Can you work these out from the model? Positions are in its coordinate system, mm. Give positions to 0.01 mm unless a question says otherwise; leave off trailing zeros. Order: outer loops, then holes, each group sorted by start corner. A loop starts at its lowest first (then second) coordinate and runs counter-clockwise, first axis right, second up. Notation, with made-up numbers: M 2.5,16 L 28.5,16 A17 ccw 28.5,41 Z; hole C -32,43.25 d8. An arc over 180 degrees is marked long. Answer as a JSON object with one key per item and string values.
Autodesk Inventor part; units mm, degrees
ref_plane "YZ Plane" through (0, 0, 0) normal (1, 0, 0) x (0, 1, 0)
ref_plane "XZ Plane" through (0, 0, 0) normal (0, 1, 0) x (-1, 0, 0)
ref_plane "XY Plane" through (0, 0, 0) normal (0, 0, 1) x (1, 0, 0)
sketch "Sketch1" plane through (0, 0, 0) normal (0, 0, 1) x (1, 0, 0)
  circle A0 centre (0, 0) radius 8.001
  dimension "d0" = 16.002
extrude "Extrusion1" add sketch "Sketch1" along normal mid plane 20.574
sketch "Sketch2" plane through (0, 0, 10.287) normal (0, 0, 1) x (1, 0, 0)
  circle A0 centre (0, 0) radius 8.001
  circle A1 centre (0, 0) radius 14.351
  dimension "d29" = 28.702
extrude "Extrusion2" add sketch "Sketch2" along normal blind 4.826 contours A0 | A1
sketch "Sketch4" plane through (0, 0, -10.287) normal (0, 0, -1) x (-1, 0, 0)
  circle A0 centre (0, 0) radius 8.001
hole "Hole2" at (0, 0, -10.287) direction (0, 0, 1) diameter 7.7978 end through all
chamfer "Chamfer1" distance 0.381 angle 45 1 edges at (-8.001, 0, -10.287)
sketch "Sketch6" plane through (0, 0, 15.113) normal (0, 0, 1) x (1, 0, 0)
  circle A0 centre (0, 0) radius 14.351
  circle A1 centre (0, 0) radius 11.4134 construction
  point P0 (0, 11.4134)
hole "Hole3" at (0, 11.4134, 15.113) direction (0, 0, -1) diameter 3.556 end through all
pattern_circular "Circular Pattern1" count 3 over 360 about axis through (0, 0, 10.287) along (0, 0, 1) of "Hole3"
properties part number "LeadScrewNut" material "ABS Plastic"
1) I'm going to push flat-ended pins straight in: pin 1 Ø1 at (x, z) = (-3, 9) entering from +Y; pin 2 Ø4 at (y, z) = (4, -2) entering from -X; pin 3 Ø6 at (y, z) = (-3, 7.5) entering from -X. Where does each tip first touch, or does it pass through?
Results found:
{"pin 1": "stops at y = 7.6", "pin 2": "stops at x = -7.75", "pin 3": "stops at x = -14.23"}
2) I want a section at A-A on y = 0. Write out the boundary of the cut face in (x, z).
Results found:
{"outline": "M -14.35,10.29 L -8,10.29 L -8,-9.91 L -7.62,-10.29 L -3.9,-10.29 L -3.9,15.11 L -14.35,15.11 Z; M 3.9,-10.29 L 7.62,-10.29 L 8,-9.91 L 8,10.29 L 14.35,10.29 L 14.35,15.11 L 3.9,15.11 Z"}
3) I want a section at B-B on x = 0. Write out the boundary of the cut face in (y, z), and give its area (3 significant figures).
Results found:
{"outline": "M -14.35,10.29 L -8,10.29 L -8,-9.91 L -7.62,-10.29 L -3.9,-10.29 L -3.9,15.11 L -14.35,15.11 Z; M 3.9,-10.29 L 7.62,-10.29 L 8,-9.91 L 8,10.29 L 9.64,10.29 L 9.64,15.11 L 3.9,15.11 Z; M 13.19,10.29 L 14.35,10.29 L 14.35,15.11 L 13.19,15.11 Z", "area": "252 mm²"}
4) Thinking about a two-plate mould opening in Y: for faces 1 (the face through (-8.15, -5.32, 12.67)), 2 (the face through (-1.73, -7.81, 0.33)), 3 (the face through (6, -6, 10.287)), which applies, pulls with the +Y half, pulls with the -Y half, needs draft (parallel to the pull), parting line crosses it, or undercut?
Results found:
{"face 1": "undercut", "face 2": "parting line crosses it", "face 3": "needs draft"}
5) I need wall thicknesses on L1, parallel to Y at x = 0, z = -4.75; L2, parallel to Z at x = -4, y = 10.5; L3, parallel to Y at x = -2.25, z = 9. Which ranges of each line are inside material? Lowest first, please.
Results found:
{"L1": "y = -8 to -3.9, 3.9 to 8", "L2": "z = 10.29 to 15.11", "L3": "y = -7.68 to -3.18, 3.18 to 7.68"}
6) I want a section at D-D on z = -2.75. Write out the boundary of the cut face in (x, y).
Results found:
{"outline": "C 0,0 d16; hole C 0,0 d7.8"}
7) I want a section at C-C on x = 9.5. Write out the boundary of the cut face in (y, z).
Results found:
{"outline": "M -10.76,10.29 L -7.44,10.29 L -7.44,15.11 L -10.76,15.11 Z; M -3.97,10.29 L 10.76,10.29 L 10.76,15.11 L -3.97,15.11 Z"}
